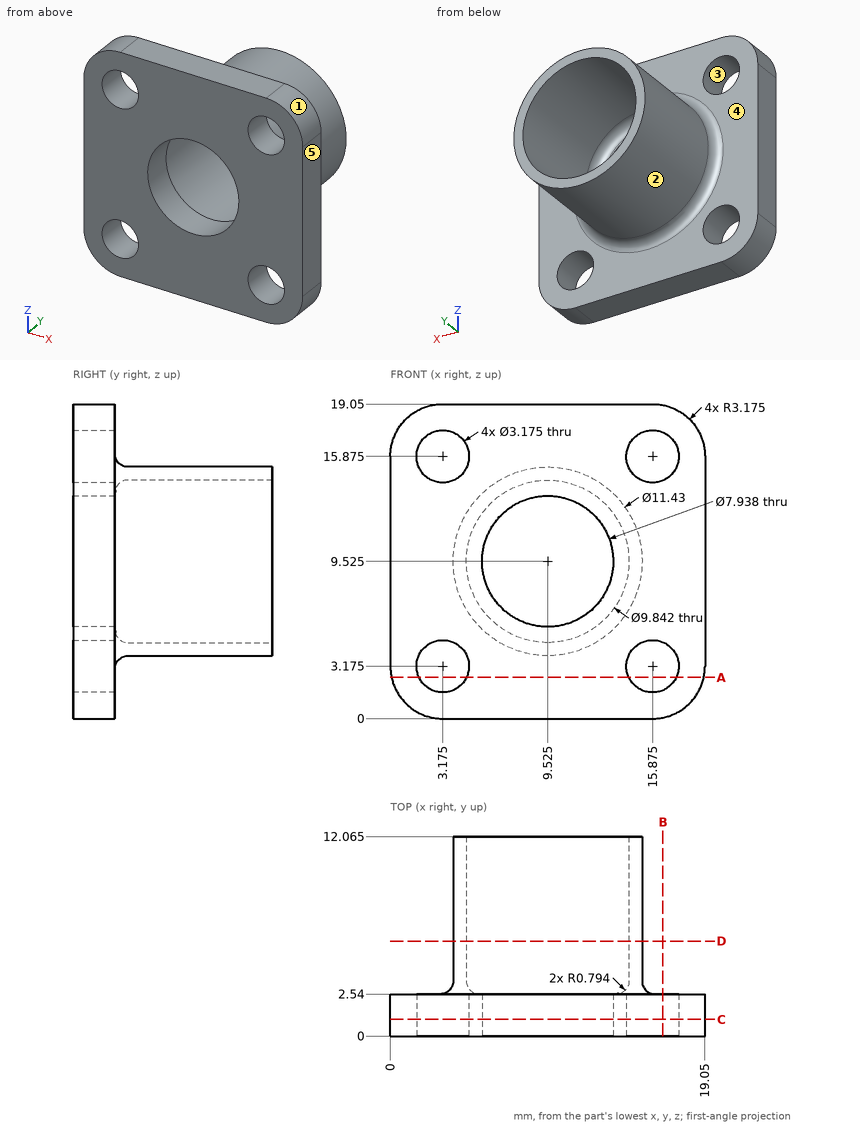
Check sheet for the drawn part. Datum: minimum x, y, z corner. Units: mm. A direction names the side the tool comes from. Round coordinates to 2 decimals unless told otherwise and drop trailing zeros. Order: outer loops, then holes, each group sorted by start corner. A loop starts at its lowest first (then second) coordinate and runs counter-clockwise, first axis right, second up.
1) Section check D-D (y = 5.75). Record the boundary of the cut face in (x, z) (1 decimal).
2) Go/stop test with flat-tipped pins: pin 1 Ø1.9 at (x, z) = (3.175, 15.875) entering from -Y; pin 2 Ø9 at (x, z) = (9.525, 9.525) entering from +Y; pin 3 Ø5 at (x, z) = (15.875, 15.875) entering from +Y; pin 4 Ø1.5 at (y, z) = (10.5, 5) entering from +X (1 decimal). Record where each tip stops, or that it passes through.
3) Section check A-A (z = 2.5). Record the boundary of the cut face in (x, y).
4) Section check B-B (x = 16.5). Record the boundary of the cut face in (y, z) (1 decimal).
5) Mould release check, pull along X, two halves, no side actions. Record for the marked faces 3, 4 and 5: +X half, -X half, draft (parallel to the pull), parting line (faces both ways), or undercut.
6) Tool access check on the marked faces 1 and 2. Record the directions out of +Z, -Z, +X, -X, +Y, -Y that give a thin tool (end or side, any length) a straight path to the whole face; none if there is none.
7) Section check C-C (y = 1). Give the number of separate pieces and of enclosed holes in the cut face, and give its area (3 significant figures).
8) Scan lines: line 1 (Z direction, x = 15.5, y = 1.25); line 2 (Z direction, x = 10, y = 6.25); line 3 (Y direction, x = 18.25, z = 4.5). Record each from-to range of solid material in increasing order.
Result:
1. outline: circle Ø11.4 at (9.5, 9.5); hole circle Ø9.8 at (9.5, 9.5)
2. pin 1: passes through
2. pin 2: stops at y = 2.63
2. pin 3: stops at y = 2.54
2. pin 4: stops at x = 13.8
3. outline: (0.07, 0) - (1.74, 0) - (1.74, 2.54) - (0.07, 2.54) - close; (4.61, 0) - (14.44, 0) - (14.44, 2.54) - (4.61, 2.54) - close; (17.31, 0) - (18.98, 0) - (18.98, 2.54) - (17.31, 2.54) - close
4. outline: (0, 0.1) - (2.5, 0.1) - (2.5, 1.7) - (0, 1.7) - close; (0, 4.6) - (2.5, 4.6) - (2.5, 14.4) - (0, 14.4) - close; (0, 17.3) - (2.5, 17.3) - (2.5, 19) - (0, 19) - close
5. face 3: undercut
5. face 4: draft
5. face 5: +X half
6. face 1: +Z, +X, +Y, -Y
6. face 2: +Y
7. separate pieces: 1
7. enclosed holes: 5
7. area: 273 mm2
8. line 1: z = 0 to 1.63, 4.72 to 14.33, 17.42 to 19.05
8. line 2: z = 3.83 to 4.63, 14.42 to 15.22
8. line 3: y = 0 to 2.54
